Source: CAD feature listing. Evaluate the final solid. Frame: model axes, mm. A direction names the side the tool comes from. Give positions to 0.01 mm unless a question says otherwise; leave off trailing zeros. Loops run counter-clockwise (first coordinate to the right, second up) from the corner with the lowest first, then second, coordinate; pieces in that order, holes last.
from build123d import *

# Parameters (mm, degrees)
SKETCH004_R      = 1
SKETCH004_W      = 24
SKETCH004_H      = 12
EXTRUDE003_DEPTH = 22
SKETCH006_W      = 39.5
SKETCH006_H      = 39.5
SKETCH006_W_2    = 37.5
SKETCH006_H_2    = 37.5
EXTRUDE004_DEPTH = 2
SKETCH003_R      = 1
SKETCH003_W      = 24
SKETCH003_H      = 12
EXTRUDE002_DEPTH = 2
FILLET001_R      = 1
CHAMFER_SIZE     = 1


with BuildPart() as extrude003:
    # Sketch004 → Extrude003 (new body)
    with BuildSketch(Plane.XY):
        with BuildLine():
            Line((34, 39), (6, 39))
            Line((6, 39), (6, 33))
            ThreePointArc((6, 33), (4, 31), (6, 29))
            Line((6, 29), (6, 23))
            Line((6, 23), (34, 23))
            Line((34, 23), (34, 29))
            ThreePointArc((34, 29), (36, 31), (34, 33))
            Line((34, 33), (34, 39))
        make_face()
        with Locations((6, 31)):
            Circle(SKETCH004_R, mode=Mode.SUBTRACT)
        with Locations((34, 31)):
            Circle(SKETCH004_R, mode=Mode.SUBTRACT)
        with Locations((20, 31)):
            Rectangle(SKETCH004_W, SKETCH004_H, mode=Mode.SUBTRACT)
    extrude(amount=-EXTRUDE003_DEPTH)


with BuildPart() as extrude004:
    # Sketch006 → Extrude004 (new body)
    with BuildSketch(Plane.XY):
        with Locations((20.25, 20.25)):
            Rectangle(SKETCH006_W, SKETCH006_H)
        with Locations((20.25, 20.25)):
            Rectangle(SKETCH006_W_2, SKETCH006_H_2, mode=Mode.SUBTRACT)
    extrude(amount=-EXTRUDE004_DEPTH)


with BuildPart() as chamfer_body:
    # Sketch003 → Extrude002 (new body)
    with BuildSketch(Plane.XY):
        with BuildLine():
            Line((0, -2), (40, -2))
            ThreePointArc((40, -2), (41.414214, -1.414214), (42, 0))
            Line((42, 0), (42, 40))
            ThreePointArc((42, 40), (41.414214, 41.414214), (40, 42))
            Line((40, 42), (0, 42))
            ThreePointArc((0, 42), (-1.414214, 41.414214), (-2, 40))
            Line((-2, 40), (-2, 0))
            ThreePointArc((-2, 0), (-1.414214, -1.414214), (0, -2))
        make_face()
        with Locations((2, 38)):
            Circle(SKETCH003_R, mode=Mode.SUBTRACT)
        with Locations((38, 38)):
            Circle(SKETCH003_R, mode=Mode.SUBTRACT)
        with Locations((20, 2)):
            Circle(SKETCH003_R, mode=Mode.SUBTRACT)
        with Locations((20, 31)):
            Rectangle(SKETCH003_W, SKETCH003_H, mode=Mode.SUBTRACT)
    extrude(amount=EXTRUDE002_DEPTH)

    # Fillet001
    fillet001_edges = [chamfer_body.edges().sort_by_distance(p)[0] for p in [
        (20, 42, 2),
    ]]
    fillet(fillet001_edges, radius=FILLET001_R)

    # Fusion001: union Extrude004
    add(extrude004.part)

    # Fusion002: union Extrude003
    add(extrude003.part)

    # Chamfer
    chamfer_edges = [chamfer_body.edges().sort_by_distance(p)[0] for p in [
        (19, 2, 2),
        (1, 38, 2),
        (37, 38, 2),
    ]]
    chamfer(chamfer_edges, length=CHAMFER_SIZE)


solid = chamfer_body.part
1) Reachability of faces 5 (the flat face through (0.5, 20, -1)), 6 (the flat face through (20, 1.5, -1)), 7 (the flat face through (20, 40, -1)), 8 (the cylindrical face through (20.924, 1.617, 0.493)), 9 (the flat face through (40, 20, -1)) from +Z, -Z, +X, -X, +Y, -Y: full face, straight path, thin tool, end or side. Return the list, or none.
Checks:
face 5: -Z, -X, +Y, -Y
face 6: -Z
face 7: -Z, +X, -X, +Y
face 8: +Z
face 9: -Z, +X, +Y, -Y
2) Ray query, probe 1 along X at (y, z) = (38, 0.6); probe 2 along X at (y, z) = (38, -1.75); probe 3 along Y at (x, z) = (20, 0.6). Return the intervals inside material, ascending.
Checks:
probe 1: x = -2 to 1, 3 to 37, 39 to 42
probe 2: x = 0.5 to 1.5, 6 to 34, 39 to 40
probe 3: y = -2 to 1, 3 to 25, 37 to 42
3) Contact query for flat-ended pins moving along their axis: P1, Ø1.2, axis at x = 20, y = 2, coming from the -Z side; P2, Ø1.5, axis at x = 37, z = -6, coming from the +Y side; P3, Ø2, axis at x = 5.5, y = 31.5, coming from the -Z side; P4, Ø4, axis at x = 16.5, y = 10.5, coming from the -Z side. Output: stop coordinate, or through.
Checks:
P1: stops at z = -2
P2: passes through
P3: stops at z = -22
P4: stops at z = 0
4) Pull-direction query (Y, two-part tool) for faces 1 (the cylindrical face through (34, 32, -11)), 2 (the flat face through (36, 39, -1)), 3 (the flat face through (19, 1, -2)), 4 (the cylindrical face through (41.4, -1.43, 0.49)); classes: released by +Y, released by -Y, zero draft, split by the parting line, or undercut.
Checks:
face 1: undercut
face 2: undercut
face 3: zero draft
face 4: released by -Y
5) Cut plane B-B (x = 16.5). Return loops of the section in (y, z), and give its area (3 significant figures).
Checks:
outline: (-2, 0) - (0.5, 0) - (0.5, -2) - (1.5, -2) - (1.5, 0) - (23, 0) - (23, -22) - (25, -22) - (25, 2) - (-1, 2) arc R1 ccw to (-2, 1) - close; (37, -22) - (39, -22) - (39, -2) - (40, -2) - (40, 0) - (42, 0) - (42, 1) arc R1 ccw to (41, 2) - (37, 2) - close
area: 156 mm2
6) Cut plane A-A (z = -16.5). Return loops of the section in (x, y).
Checks:
outline: (6, 23) - (34, 23) - (34, 29) arc R2 ccw to (34, 33) - (34, 39) - (6, 39) - (6, 33) arc R2 ccw to (6, 29) - close; hole circle Ø2 at (6, 31); hole (8, 25) - (32, 25) - (32, 37) - (8, 37) - close; hole circle Ø2 at (34, 31)
7) Cut plane D-D (y = 5.5). Return loops of the section in (x, z).
Checks:
outline: (-2, 0) - (0.5, 0) - (0.5, -2) - (1.5, -2) - (1.5, 0) - (39, 0) - (39, -2) - (40, -2) - (40, 0) - (42, 0) - (42, 1) arc R1 ccw to (41, 2) - (-1, 2) arc R1 ccw to (-2, 1) - close
